Autodesk Inventor part; units mm, degrees
ref_plane "YZ Plane" through (0, 0, 0) normal (1, 0, 0) x (0, 1, 0)
ref_plane "XZ Plane" through (0, 0, 0) normal (0, 1, 0) x (-1, 0, 0)
ref_plane "XY Plane" through (0, 0, 0) normal (0, 0, 1) x (1, 0, 0)
sketch "Sketch1" plane through (0, 0, 0) normal (0, 1, 0) x (-1, 0, 0)
  line L0 (-7.5, 15) -> (7.5, 15)
  line L1 (7.5, 15) -> (7.5, -15)
  line L2 (7.5, -15) -> (-7.5, -15)
  line L3 (-7.5, -15) -> (-7.5, 15)
  line L4 (-7.5, 15) -> (7.5, -15) construction
  line L5 (7.5, 15) -> (-7.5, -15) construction
  point P0 (0, 0)
  dimension "d0" = 15
  dimension "d1" = 30
extrude "Extrusion1" add sketch "Sketch1" along normal blind 4
chamfer "Chamfer1" distance 2.5 distance2 1 1 edges at (7.5, 2, -15) measured on face at (7.5, 1.3333, 5)
chamfer "Chamfer2" distance 1 distance2 2.5 1 edges at (-7.5, 2, -15) measured on face at (1.8333, 2.6667, -15)
sketch "Sketch3" plane through (0, 0, 0) normal (0, -1, 0) x (1, 0, 0)
  line L0 (0, 0) -> (4, 0)
  line L1 (0, 0) -> (-4, 0)
  dimension "d14" = 4
  dimension "d15" = 4
hole "Hole1" at (4, 0, 0) at (-4, 0, 0) direction (0, 1, 0) diameter 2.1565 depth 2
sketch "Sketch4" plane through (0, 0, 0) normal (0, -1, 0) x (1, 0, 0)
  line L0 (7.5, 15) -> (7.5, -12.5)
  line L1 (7.5, -12.5) -> (7.5, -7.5)
  line L2 (7.5, -7.5) -> (2.5, -7.5)
  line L3 (2.5, -7.5) -> (2.5, -5.5)
  line L4 (2.5, -5.5) -> (-2.5, -5.5)
  line L5 (-2.5, -5.5) -> (-2.5, -7.5)
  line L6 (-2.5, -7.5) -> (-7.5679, -7.5)
  line L7 (-7.5679, -7.5) -> (-7.5679, -12.5)
  line L8 (6.5, -15) -> (-6.5, -15)
  line L9 (-7.5679, -12.5) -> (-6.5, -15)
  line L10 (7.5, -12.5) -> (6.5, -15)
  line L11 (-6.5, -15) -> (6.5, -15)
  line L12 (6.5, -15) -> (7.5, -12.5)
  point P0 (0, 0)
  dimension "d23" = 5
  dimension "d24" = 5
  dimension "d25" = 2
  dimension "d26" = 5
split body "Split1" sketch "Sketch4" result one side removed curves L2 L3 L4 L5 L6 L7 L9 L11 L12 L1 removed pieces at (0.8333, 0.5, -12.5)
sketch "Sketch5" plane through (0, 4, 0) normal (0, 1, 0) x (1, 0, 0)
  line L0 (-7.5, 7.5) -> (-7.5, -15)
  line L1 (7.5, -15) -> (7.5, 7.5)
  line L2 (-7.5, -15) -> (7.5, -15)
  line L3 (7.5, -15) -> (7.5, -10)
  line L4 (7.5, -10) -> (-7.5, -10)
  line L5 (-7.5, -10) -> (-7.5, -15)
  point P0 (0, 0)
  dimension "d27" = 5
extrude "Extrusion3" add sketch "Sketch5" along normal blind 6 and the other way blind 10
sketch "Sketch6" plane through (7.5, 0, -7.5) normal (1, 0, 0) x (0, 0, -1)
  line L0 (0, 4) -> (0, 0)
  line L1 (0, 2) -> (-3, 2)
  line L2 (-17.5, 2) -> (-14.5, 2)
  point P0 (-7.5, 0)
  dimension "d38" = 3
  dimension "d39" = 3
hole "Hole2" at (7.5, 2, 7) at (7.5, 2, -4.5) direction (-1, 0, 0) diameter 1.1811 depth 3
sketch "Sketch7" plane through (-7.5, 0, -7.5) normal (-1, 0, 0) x (0, 0, 1)
  circle A0 centre (3, 2) radius 0.5906
  circle A1 centre (14.5, 2) radius 0.5906
  point P0 (7.5, 0)
hole "Hole3" at (-7.5, 2, 7) at (-7.5, 2, -4.5) direction (1, 0, 0) diameter 1.1811 depth 3
sketch "Sketch8" plane through (0, -6, 0) normal (0, -1, 0) x (1, 0, 0)
  line L0 (7.5, 10) -> (7.5, 15)
  line L1 (7.5, 12.5) -> (4, 12.5)
  line L2 (-7.5, 10) -> (-7.5, 15)
  line L3 (-7.5, 12.5) -> (-4, 12.5)
  point P0 (0, 0)
  dimension "d54" = 3.5
  dimension "d55" = 3.5
hole "Hole4" at (4, -6, 12.5) at (-4, -6, 12.5) direction (0, 1, 0) diameter 2.1565 depth 3
properties part number "copper_thermal_contact" material "Copper"
Part model, mm, in its own coordinate system. A direction names the side the tool comes from. Coordinates: 2 decimals unless noted, no trailing zeros. Order: outer loops, then holes, each group sorted by start corner. A loop starts at its lowest first (then second) coordinate and runs counter-clockwise, first axis right, second up.
(1) Probe L1, parallel to X at y = 1.4, z = 0; L2, parallel to Z at x = -6.1, y = 2; L3, parallel to Y at x = 5.55, z = 7. List the from-to ranges inside material, lowest first.
Check sheet entries:
L1: x = -7.5 to -5.08, -2.92 to 2.92, 5.08 to 7.5
L2: z = -7.5 to -5.09, -3.91 to 6.41, 7.59 to 15
L3: y = 0 to 1.41, 2.59 to 4
(2) Pull direction Y, two halves, no side cores. Call faces 1 (the face through (5.979, 2.226, 6.454)), 2 (the face through (-4, -3, 13)), 3 (the face through (5, 2, -7.5)): pulls with the +Y half, pulls with the -Y half, needs draft (parallel to the pull), parting line crosses it, or undercut.
Check sheet entries:
face 1: undercut
face 2: pulls with the -Y half
face 3: needs draft
(3) Pin check, flat tips, straight feed: pin 1 Ø1.3 at (x, z) = (-4, 0) entering from -Y; pin 2 Ø1.1 at (y, z) = (2, 7) entering from +X; pin 3 Ø5 at (x, z) = (1, 1.5) entering from -Y. Stop position of each tip, or through.
Check sheet entries:
pin 1: stops at y = 2
pin 2: stops at x = 4.5
pin 3: stops at y = 0
(4) Slice it at A-A, the plane z = 7. Write the cut outline in (x, y).
Check sheet entries:
outline: (-7.5, 0) - (7.5, 0) - (7.5, 1.41) - (4.5, 1.41) - (4.5, 2.59) - (7.5, 2.59) - (7.5, 4) - (-7.5, 4) - (-7.5, 2.59) - (-4.5, 2.59) - (-4.5, 1.41) - (-7.5, 1.41) - close
(5) Slice it at D-D, the plane y = 5. Write the cut outline in (x, z).
Check sheet entries:
outline: (-7.5, 10) - (7.5, 10) - (7.5, 15) - (-7.5, 15) - close
(6) Slice it at B-B, the plane y = -4.5. Write the cut outline in (x, z).
Check sheet entries:
outline: (-7.5, 10) - (7.5, 10) - (7.5, 15) - (-7.5, 15) - close; hole circle Ø2.16 at (-4, 12.5); hole circle Ø2.16 at (4, 12.5)
(7) Slice it at C-C, the plane x = 4. Write the cut outline in (y, z).
Check sheet entries:
outline: (-6, 10) - (0, 10) - (0, 1.08) - (2, 1.08) - (2, -1.08) - (0, -1.08) - (0, -7.5) - (4, -7.5) - (4, 10) - (10, 10) - (10, 15) - (-6, 15) - (-6, 13.58) - (-3, 13.58) - (-3, 11.42) - (-6, 11.42) - close
(8) Tool access for faces 4 (the face through (4.5, 2, -4.5)), 5 (the face through (-5.979, 2.226, 7.546)), 6 (the face through (0, 2, -5.5)), 7 (the face through (-3.6, -4.5, 11.5)), 8 (the face through (0, -3, 10)): list every direction of +Z, -Z, +X, -X, +Y, -Y with a clear straight run to the whole face (end or side of a thin tool).
Check sheet entries:
face 4: +X
face 5: -X
face 6: -Z, +Y, -Y
face 7: -Y
face 8: -Z, +X, -X, -Y
